Check sheet for the modelled part. Datum: model origin and axes. Units: mm. A direction names the side the tool comes from. Give positions to 0.01 mm unless a question says otherwise; leave off trailing zeros. Loops run counter-clockwise (first coordinate to the right, second up) from the corner with the lowest first, then second, coordinate; pieces in that order, holes last. Notation, with made-up numbers: M 88,36 L 137,36 A26 ccw 137,50 Z; hole C 41,6 d11. An arc over 180 degrees is marked long. Use one line per item in the form item = value.
from build123d import *

# Parameters (mm, degrees)
BOSS_EXTRUDE4_DEPTH = 11.999999999999996
BOSS_EXTRUDE5_DEPTH = 3.5
BOSS_EXTRUDE6_DEPTH = 12
CUT_EXTRUDE2_DEPTH  = 8.5
BOSS_EXTRUDE7_DEPTH = 3.5000000000000004
SKETCH2_R           = 8.1
CUT_EXTRUDE3_DEPTH  = 12
FILLET1_R           = 5
FILLET2_R           = 2
SKETCH3_R           = 2.2499999999999964
CUT_EXTRUDE4_DEPTH  = 12
SKETCH4_R           = 9.500000000000002
SKETCH4_R_2         = 8.000000000000002
SKETCH4_R_3         = 9.499999999999995
SKETCH4_R_4         = 7.999999999999998
BOSS_EXTRUDE8_DEPTH = 20


with BuildPart() as part:
    # Sketch1 → Boss-Extrude4 (new body)
    with BuildSketch(Plane(origin=(0, 0, 0), x_dir=(1, 0, 0), z_dir=(0, 1, 0))):
        with BuildLine():
            ThreePointArc((-105.23956914411866, 60.05130546378884), (-126.31086817026393, 62.500868149406244), (-128.76043085588134, 41.429569123260976))
            ThreePointArc((-128.76043085588134, 41.42956912326096), (-78.3921989201775, 0.4513014224205847), (-15.424890802752289, -15.400995588922257))
            ThreePointArc((-15.424890802752284, -15.400995588922251), (-20.878753235246265, -0.5691494549701637), (-16.67921047602729, 14.665420305521598))
            ThreePointArc((-16.679210476027265, 14.665420305521593), (-65.8857769449076, 27.74562513419724), (-105.23956914411866, 60.05130546378885))
        make_face()
    extrude(amount=BOSS_EXTRUDE4_DEPTH)

    # Sketch1_6 → Boss-Extrude5 (add)
    with BuildSketch(Plane(origin=(0, 0, 0), x_dir=(1, 0, 0), z_dir=(0, 1, 0))):
        with BuildLine():
            ThreePointArc((-16.67921047602729, 14.665420305521598), (-20.878753235246265, -0.5691494549701637), (-15.424890802752284, -15.400995588922251))
            ThreePointArc((-15.424890802752289, -15.400995588922257), (-7.086372530747029, -15.406529466177687), (1.2395691441186596, -14.94869453621115))
            ThreePointArc((1.2395691441186607, -14.948694536211157), (14.948694536211152, 1.2395691441186514), (-1.2395691441186483, 14.948694536211152))
            ThreePointArc((-1.2395691441186347, 14.94869453621115), (-8.954828429393212, 14.55844291928571), (-16.679210476027265, 14.665420305521593))
        make_face()
    extrude(amount=BOSS_EXTRUDE5_DEPTH)

    # Sketch1_8 → Boss-Extrude6 (add)
    with BuildSketch(Plane(origin=(0, 0, 0), x_dir=(1, 0, 0), z_dir=(0, 1, 0))):
        with BuildLine():
            ThreePointArc((-16.67921047602729, 14.665420305521598), (-20.878753235246265, -0.5691494549701637), (-15.424890802752284, -15.400995588922251))
            ThreePointArc((-15.424890802752289, -15.400995588922257), (-7.086372530747029, -15.406529466177687), (1.2395691441186596, -14.94869453621115))
            ThreePointArc((1.2395691441186607, -14.948694536211157), (14.948694536211152, 1.2395691441186514), (-1.2395691441186483, 14.948694536211152))
            ThreePointArc((-1.2395691441186347, 14.94869453621115), (-8.954828429393212, 14.55844291928571), (-16.679210476027265, 14.665420305521593))
        make_face()
    extrude(amount=BOSS_EXTRUDE6_DEPTH)

    # Sketch1_9 → Cut-Extrude2 (cut)
    with BuildSketch(Plane(origin=(0, 0, 0), x_dir=(1, 0, 0), z_dir=(0, 1, 0))):
        with BuildLine():
            ThreePointArc((-16.67921047602729, 14.665420305521598), (-20.878753235246265, -0.5691494549701637), (-15.424890802752284, -15.400995588922251))
            ThreePointArc((-15.424890802752289, -15.400995588922257), (-7.086372530747029, -15.406529466177687), (1.2395691441186596, -14.94869453621115))
            ThreePointArc((1.2395691441186607, -14.948694536211157), (14.948694536211152, 1.2395691441186514), (-1.2395691441186483, 14.948694536211152))
            ThreePointArc((-1.2395691441186347, 14.94869453621115), (-8.954828429393212, 14.55844291928571), (-16.679210476027265, 14.665420305521593))
        make_face()
    extrude(amount=CUT_EXTRUDE2_DEPTH, mode=Mode.SUBTRACT)

    # Sketch1_10 → Boss-Extrude7 (add)
    with BuildSketch(Plane(origin=(0, 0, 0), x_dir=(1, 0, 0), z_dir=(0, 1, 0))):
        with BuildLine():
            ThreePointArc((-16.67921047602729, 14.665420305521598), (-20.878753235246265, -0.5691494549701637), (-15.424890802752284, -15.400995588922251))
            ThreePointArc((-15.424890802752289, -15.400995588922257), (-7.086372530747029, -15.406529466177687), (1.2395691441186596, -14.94869453621115))
            ThreePointArc((1.2395691441186607, -14.948694536211157), (14.948694536211152, 1.2395691441186514), (-1.2395691441186483, 14.948694536211152))
            ThreePointArc((-1.2395691441186347, 14.94869453621115), (-8.954828429393212, 14.55844291928571), (-16.679210476027265, 14.665420305521593))
        make_face()
    extrude(amount=BOSS_EXTRUDE7_DEPTH)

    # Sketch2 → Cut-Extrude3 (cut)
    with BuildSketch(Plane(origin=(0, 11.999999999999996, 0), x_dir=(1, 0, 0), z_dir=(0, 1, 0))):
        with Locations(Location((0, 0, 0), (0, 0, 270))):
            Circle(SKETCH2_R)
    extrude(amount=-CUT_EXTRUDE3_DEPTH, mode=Mode.SUBTRACT)

    # Fillet1
    fillet1_edges = [part.edges().sort_by_distance(p)[0] for p in [
        (-16.67921047602728, 6, -14.665420305521597),
    ]]
    fillet(fillet1_edges, radius=FILLET1_R)

    # Fillet2
    fillet2_edges = [part.edges().sort_by_distance(p)[0] for p in [
        (-15.424890802752289, 6, 15.400995588922266),
    ]]
    fillet(fillet2_edges, radius=FILLET2_R)

    # Sketch3 → Cut-Extrude4 (cut)
    with BuildSketch(Plane(origin=(0, 11.999999999999996, 0), x_dir=(1, 0, 0), z_dir=(0, 1, 0))):
        with Locations(Location((-107.81660725396851, 54.30249040498051, 0), (0, 0, 270))):
            Circle(SKETCH3_R)
        with Locations(Location((-112.49908312253997, 48.44378579216329, 0), (0, 0, 270))):
            Circle(SKETCH3_R)
    extrude(amount=-CUT_EXTRUDE4_DEPTH, mode=Mode.SUBTRACT)

    # Sketch4 → Boss-Extrude8 (add)
    # profile 1 of 2: a face of its own
    with BuildSketch(Plane(origin=(0, 11.999999999999996, 0), x_dir=(1, 0, 0), z_dir=(0, 1, 0))):
        with Locations(Location((-35.824132830362714, 1.9278264844930209, 0), (0, 0, 270))):
            Circle(SKETCH4_R)
        with Locations(Location((-35.824132830362714, 1.9278264844930209, 0), (0, 0, 270))):
            Circle(SKETCH4_R_2, mode=Mode.SUBTRACT)
    # profile 2 of 2: a face of its own
    with BuildSketch(Plane(origin=(0, 11.999999999999996, 0), x_dir=(1, 0, 0), z_dir=(0, 1, 0))):
        with Locations(Location((-82.24716798080135, 19.60428986869888, 0), (0, 0, 270))):
            Circle(SKETCH4_R_3)
        with Locations(Location((-82.24716798080135, 19.60428986869888, 0), (0, 0, 270))):
            Circle(SKETCH4_R_4, mode=Mode.SUBTRACT)
    extrude(amount=BOSS_EXTRUDE8_DEPTH)


solid = part.part
1) Depth check by flat-ended pin: pin 1 Ø7 at (x, z) = (-107.82, -54.3) entering from -Y; pin 2 Ø2 at (y, z) = (6, -42) entering from -X; pin 3 Ø5 at (x, y) = (-10, 11) entering from -Z; pin 4 Ø5 at (x, z) = (-82, -16.5) entering from +Y. Enter the tip coordinate at first touch or a pass-through.
Evaluation:
pin_1 = 0
pin_2 = -129.85
pin_3 = -14.59
pin_4 = 12
2) Section check D-D (x = -31.5). Record the cut outline in (y, z).
Evaluation:
outline = M 0,-16.28 L 12,-16.28 L 12,-10.39 L 32,-10.39 L 32,-8.66 L 12,-8.66 L 12,4.8 L 32,4.8 L 32,6.53 L 12,6.53 L 12,14.08 L 0,14.08 Z
3) Section check A-A (z = 0). Record the cut outline in (x, y).
Evaluation:
outline = M -77.48,0 L -8.1,0 L -8.1,3.5 L -20.9,3.5 L -20.9,8.5 L -8.1,8.5 L -8.1,12 L -26.52,12 L -26.52,32 L -28.06,32 L -28.06,12 L -43.59,12 L -43.59,32 L -45.13,32 L -45.13,12 L -77.48,12 Z; M 8.1,0 L 15,0 L 15,3.5 L 8.1,3.5 Z; M 8.1,8.5 L 15,8.5 L 15,12 L 8.1,12 Z
4) Release check for a two-part mould opening along X. For faces 1 (the face through (-20.792, 5.965, 1.864)), 2 (the face through (-82, 12, -20)), 3 (the face through (-9, 3.5, 0)) record: pulls with the +X half, pulls with the -X half, needs draft (parallel to the pull), parting line crosses it, or undercut.
Evaluation:
face_1 = pulls with the +X half
face_2 = undercut
face_3 = needs draft
5) Set-up check for faces 4 (the face through (-126.05, 5.916, -62.703)), 5 (the face through (-45.098, 21.86, -3.987)): record each of +Z, -Z, +X, -X, +Y, -Y from which the full face is reachable in a straight line by a thin tool's end or side.
Evaluation:
face_4 = +Y, -Y
face_5 = +Y
6) Scan lines: line 1 (Y direction, x = -5.5, z = 7.5); line 2 (X direction, y = 16.5, z = -19); line 3 (Y direction, x = -119, z = -37.5). Record each from-to range of solid material in increasing order.
Evaluation:
line_1 = 0 to 3.5, 8.5 to 12
line_2 = -91.73 to -90.22, -74.27 to -72.77
line_3 = 0 to 12
7) Section check B-B (x = 4.5). Record the cut outline in (y, z), then the cut area to 3 significant figures.
Evaluation:
outline = M 0,-14.31 L 3.5,-14.31 L 3.5,-6.73 L 0,-6.73 Z; M 0,6.73 L 3.5,6.73 L 3.5,14.31 L 0,14.31 Z; M 8.5,-14.31 L 12,-14.31 L 12,-6.73 L 8.5,-6.73 Z; M 8.5,6.73 L 12,6.73 L 12,14.31 L 8.5,14.31 Z
area = 106 mm^2
8) Section check C-C (y = 27). Record the cut outline in (x, z).
Evaluation:
outline = C -82.25,-19.6 d19; C -35.82,-1.93 d19; hole C -82.25,-19.6 d16; hole C -35.82,-1.93 d16
